Verification items for the finished model (mm, model axes). A direction names the side the tool comes from. Round coordinates to 2 decimals unless told otherwise and drop trailing zeros. Order: outer loops, then holes, each group sorted by start corner. A loop starts at its lowest first (then second) coordinate and runs counter-clockwise, first axis right, second up. Notation, with made-up numbers: (-4, 65) -> (48, 65) arc R29 ccw to (48, 101) -> close; hole circle Ø11 at (-25.75, 60). An arc over 180 degrees is marked (long way). Return JSON: item names as keys, results as strings. Group by question number.
1) Section check A-A on z = -17. Enter the section's corners in (x, y), plus the area to 3 significant figures.
2) Section check D-D on x = -63.5. Enter the section's corners in (y, z).
3) Scan lines: L1, parallel to Y at x = 126, z = -11; L2, parallel to Z at x = -30.5, y = -69; L3, parallel to X at y = -359, z = -20.5. Record each from-to range of solid material in increasing order.
4) Section check B-B on x = 117. Enter the section's corners in (y, z).
5) Draft check along Y on faces 1 (the flat face through (-129, -25.4, -12)), 2 (the flat face through (125.91, -368.12, -15.42)), 3 (the flat face through (-1, 0, 0)). Enter one of: pulls with the +Y half, pulls with the -Y half, needs draft (parallel to the pull), parting line crosses it, or undercut.
6) Section check C-C on y = -202.5. Enter the section's corners in (x, z), plus the area to 3 significant figures.
7) Depth check by flat-ended pin: pin 1 (7.5 mm diameter, centred on x = 126, z = -21, fed in from -Y). Enter the tip coordinate at first touch or a pass-through.
8) Tool access check on faces 4 (the flat face through (128, -25.4, -12)), 5 (the flat face through (125.91, -12.52, -15.42)), 6 (the flat face through (-2, -188, -2.54)). Record the directions out of +Z, -Z, +X, -X, +Y, -Y that give a thin tool (end or side, any length) a straight path to the whole face; none if there is none.
```python
from build123d import *

# Parameters (mm, degrees)
F0_W     = 276.86
F0_H     = 5.08
F1_DEPTH = 381
F2_W     = 25.4
F2_H     = 25.4
F3_DEPTH = 25.4
F4_SIZE  = 25.39999
F5_SIZE  = 25.39999


# Not quite as in the source:
# - a fillet or chamfer is up to 0.001 mm smaller than in the source, because OpenCascade refuses the exact size


with BuildPart() as f1:
    # F0 (on Front) → F1 (new body)
    with BuildSketch(Plane.XZ):
        Rectangle(F0_W, F0_H)
    extrude(amount=F1_DEPTH)

    # F2 (on face) → F3 (join)
    with BuildSketch(Plane(origin=(0, 0, -2.54), x_dir=(1, 0, 0), z_dir=(0, 0, -1))):
        with Locations((125.73, 368.3)):
            Rectangle(F2_W, F2_H)
        with Locations((-125.73, 368.3)):
            Rectangle(F2_W, F2_H)
        with Locations((-125.73, 12.7)):
            Rectangle(F2_W, F2_H)
        with Locations((125.73, 12.7)):
            Rectangle(F2_W, F2_H)
    extrude(amount=F3_DEPTH)

    # F4 (size 25.4 in the source; OpenCascade refuses exactly that, so slightly less here)
    f4_edges = [f1.edges().sort_by_distance(p)[0] for p in [
        (-113.03, -368.3, -27.94),
    ]]
    chamfer(f4_edges, length=F4_SIZE)

    # F5 (size 25.4 in the source; OpenCascade refuses exactly that, so slightly less here)
    f5_edges = [f1.edges().sort_by_distance(p)[0] for p in [
        (113.03, -368.3, -27.94),
        (113.03, -12.7, -27.94),
        (-113.03, -12.7, -27.94),
    ]]
    chamfer(f5_edges, length=F5_SIZE)


solid = f1.part
```
Check result:
{
 "1": {"outline": "(-138.43, -381) -> (-127.49, -381) -> (-127.49, -355.6) -> (-138.43, -355.6) -> close; (-138.43, -25.4) -> (-127.49, -25.4) -> (-127.49, 0) -> (-138.43, 0) -> close; (127.49, -381) -> (138.43, -381) -> (138.43, -355.6) -> (127.49, -355.6) -> close; (127.49, -25.4) -> (138.43, -25.4) -> (138.43, 0) -> (127.49, 0) -> close", "area": "1,110 mm^2"},
 "2": {"outline": "(-381, -2.54) -> (0, -2.54) -> (0, 2.54) -> (-381, 2.54) -> close"},
 "3": {"L1": "-381 to -355.6, -25.4 to 0", "L2": "-2.54 to 2.54", "L3": "-138.43 to -130.99, 130.99 to 138.43"},
 "4": {"outline": "(-381, -6.51) -> (-355.6, -6.51) -> (-355.6, -2.54) -> (-25.4, -2.54) -> (-25.4, -6.51) -> (0, -6.51) -> (0, 2.54) -> (-381, 2.54) -> close"},
 "5": {"face 1": "undercut", "face 2": "needs draft", "face 3": "pulls with the +Y half"},
 "6": {"outline": "(-138.43, -2.54) -> (138.43, -2.54) -> (138.43, 2.54) -> (-138.43, 2.54) -> close", "area": "1,410 mm^2"},
 "7": {"pin 1": "through"},
 "8": {"face 4": "-Z, +X, -X", "face 5": "-Z, +Y, -Y", "face 6": "-Z"}
}
